```python
from build123d import *

# Parameters (mm, degrees)
SKETCH_1_W          = 32
SKETCH_1_H          = 10
EXTRUDE_1_DEPTH     = 4.5
SKETCH_2_R          = 2.1
CUT_EXTRUDE_1_DEPTH = 34.826764551
EXTRUDE_2_DEPTH     = 4
CHAMFER_1_SIZE      = 3
SKETCH_5_R          = 1.1
CUT_EXTRUDE_2_DEPTH = 34.826764551


with BuildPart() as part:
    # Эскиз1 → Бобышка-Вытянуть1 (new body)
    with BuildSketch(Plane.XY):
        with Locations((16, 5)):
            Rectangle(SKETCH_1_W, SKETCH_1_H)
    extrude(amount=EXTRUDE_1_DEPTH)

    # Эскиз2 → Вырез-Вытянуть1 (cut, through all)
    with BuildSketch(Plane(origin=(0, 10, 0), x_dir=(1, 0, 0), z_dir=(0, 1, 0))):
        with Locations((8.575, -5)):
            Circle(SKETCH_2_R)
        with Locations((23.425, -5)):
            Circle(SKETCH_2_R)
    extrude(amount=-CUT_EXTRUDE_1_DEPTH, mode=Mode.SUBTRACT)

    # Эскиз4 → Бобышка-Вытянуть2 (add)
    with BuildSketch(Plane.XZ.offset(-6)):
        with BuildLine():
            Line((6.535392195, 4.5), (7.055131585, 4.5))
            ThreePointArc((7.055131585, 4.5), (8.575, 3.4), (10.094868415, 4.5))
            Line((10.094868415, 4.5), (10.614607805, 4.5))
            ThreePointArc((10.614607805, 4.5), (8.575, 2.9), (6.535392195, 4.5))
        make_face()
        with BuildLine():
            Line((21.385392195, 4.5), (21.905131585, 4.5))
            ThreePointArc((21.905131585, 4.5), (23.425, 3.4), (24.944868415, 4.5))
            Line((24.944868415, 4.5), (25.464607805, 4.5))
            ThreePointArc((25.464607805, 4.5), (23.425, 2.9), (21.385392195, 4.5))
        make_face()
    extrude(amount=EXTRUDE_2_DEPTH)

    # Фаска1
    chamfer_1_edges = [part.edges().sort_by_distance(p)[0] for p in [
        (0, 5, 0),
        (32, 5, 0),
    ]]
    chamfer(chamfer_1_edges, length=CHAMFER_1_SIZE)

    # Эскиз5 → Вырез-Вытянуть2 (cut, through all)
    with BuildSketch(Plane(origin=(0, 0, 0), x_dir=(-1, 0, 0), z_dir=(0, 0, -1))):
        with Locations((-28.5, 5)):
            Circle(SKETCH_5_R)
        with Locations((-16, 5)):
            Circle(SKETCH_5_R)
        with Locations((-3.5, 5)):
            Circle(SKETCH_5_R)
    extrude(amount=-CUT_EXTRUDE_2_DEPTH, mode=Mode.SUBTRACT)

    # Фаска2: read off the stored shape, not the designer's step
    # Фаска2: loft between two sections, ruled curve by curve
    chamfer_2_from = [
        Edge.make_three_point_arc((3.288461538, 6.079468146, 1.5), (4.579468146, 5.211538462, 1.5), (3.711538462, 3.920531854, 1.5)),
        Edge.make_three_point_arc((3.711538462, 3.920531854, 1.5), (2.420531854, 4.788461538, 1.5), (3.288461538, 6.079468146, 1.5)),
    ]
    chamfer_2_to = [
        Edge.make_three_point_arc((2.999999479, 7.551472823, -2.709e-06), (6.051472823, 5.500000521, -2.709e-06), (4.000000521, 2.448527177, -2.709e-06)),
        Edge.make_three_point_arc((4.000000521, 2.448527177, -2.709e-06), (0.948527177, 4.499999479, -2.709e-06), (2.999999479, 7.551472823, -2.709e-06)),
    ]
    chamfer_2 = Solid(Shell([*[Face.make_surface_from_curves(chamfer_2_from[k], chamfer_2_to[k]) for k in range(2)], Face(Wire(chamfer_2_from)), Face(Wire(chamfer_2_to))]))
    add(chamfer_2, mode=Mode.SUBTRACT)

    # Chamfer 2 2: loft between two sections, ruled curve by curve
    chamfer_2_2_from = [
        Edge.make_three_point_arc((17.1, 5, 1.5), (16, 3.9, 1.5), (14.9, 5, 1.5)),
        Edge.make_three_point_arc((14.9, 5, 1.5), (16, 6.1, 1.5), (17.1, 5, 1.5)),
    ]
    chamfer_2_2_to = [
        Edge.make_three_point_arc((18.6, 5, 0), (16, 2.4, 0), (13.4, 5, 0)),
        Edge.make_three_point_arc((13.4, 5, 0), (16, 7.6, 0), (18.6, 5, 0)),
    ]
    chamfer_2_2 = Solid(Shell([*[Face.make_surface_from_curves(chamfer_2_2_from[k], chamfer_2_2_to[k]) for k in range(2)], Face(Wire(chamfer_2_2_from)), Face(Wire(chamfer_2_2_to))]))
    add(chamfer_2_2, mode=Mode.SUBTRACT)

    # Chamfer 2 3: loft between two sections, ruled curve by curve
    chamfer_2_3_from = [
        Edge.make_three_point_arc((28.711538462, 3.920531854, 1.5), (27.420531854, 4.788461538, 1.5), (28.288461538, 6.079468146, 1.5)),
        Edge.make_three_point_arc((28.288461538, 6.079468146, 1.5), (29.579468146, 5.211538462, 1.5), (28.711538462, 3.920531854, 1.5)),
    ]
    chamfer_2_3_to = [
        Edge.make_three_point_arc((29.000000521, 2.448527177, -2.709e-06), (25.948527177, 4.499999479, -2.709e-06), (27.999999479, 7.551472823, -2.709e-06)),
        Edge.make_three_point_arc((27.999999479, 7.551472823, -2.709e-06), (31.051472823, 5.500000521, -2.709e-06), (29.000000521, 2.448527177, -2.709e-06)),
    ]
    chamfer_2_3 = Solid(Shell([*[Face.make_surface_from_curves(chamfer_2_3_from[k], chamfer_2_3_to[k]) for k in range(2)], Face(Wire(chamfer_2_3_from)), Face(Wire(chamfer_2_3_to))]))
    add(chamfer_2_3, mode=Mode.SUBTRACT)


solid = part.part
```
Input: part model. Units: mm. Frame: model coordinates. A direction names the side the tool comes from. Give positions to 0.01 mm unless a question says otherwise; leave off trailing zeros. Order: outer loops, then holes, each group sorted by start corner. A loop starts at its lowest first (then second) coordinate and runs counter-clockwise, first axis right, second up. Notation, with made-up numbers: M 49,11.25 L 86,11.25 A25 ccw 86,40.25 Z; hole C -9,38.25 d9. An arc over 180 degrees is marked long. Return JSON: item names as keys, results as strings.
Item 1: Cut plane B-B (y = 1). Return loops of the section in (x, z) (3 decimals).
Solutions:
{"outline": "M 0,3 L 3,0 L 29,0 L 32,3 L 32,4.5 L 25.465,4.5 A2.1 cw 21.385,4.5 L 10.615,4.5 A2.1 cw 6.535,4.5 L 0,4.5 Z"}
Item 2: Ray query, probe 1 along X at (y, z) = (5, 3.1); probe 2 along Y at (x, z) = (3.5, 2.6); probe 3 along X at (y, z) = (4.75, 1.2). Return the intervals inside material, ascending.
Solutions:
{"probe 1": "0 to 2.4, 4.6 to 14.9, 17.1 to 27.4, 29.6 to 32", "probe 2": "0 to 3.9, 6.1 to 10", "probe 3": "1.8 to 2.12, 4.88 to 14.62, 17.38 to 27.12, 29.88 to 30.2"}
Item 3: Cut plane D-D (x = 9). Return loops of the section in (y, z).
Solutions:
{"outline": "M 0,0 L 10,0 L 10,2.94 L 6,2.94 L 6,3.46 L 2,3.46 L 2,2.94 L 0,2.94 Z"}
Item 4: Cut plane C-C (z = 1.8). Return loops of the section in (x, y), then the cut area to 3 significant figures.
Solutions:
{"outline": "M 1.2,0 L 30.8,0 L 30.8,10 L 1.2,10 Z; hole C 3.5,5 d2.2; hole C 16,5 d2.2; hole C 28.5,5 d2.2", "area": "285 mm^2"}
Item 5: Cut plane A-A (z = 3.7). State how many separate pieces and enclosed holes the cut face has, then the cut area to 3 significant figures.
Solutions:
{"separate pieces": "3", "enclosed holes": "3", "area": "254 mm^2"}
Item 6: First-contact query: P1, Ø3.5, axis at x = 28.5, y = 5, coming from the -Z side; P2, Ø0.5, axis at x = 23, z = 3.5, coming from the -Y side; P3, Ø1.3, axis at x = 9, z = 4, coming from the +Y side. Flat tips, straight axial feed; report the tip coordinate or a pass-through.
Solutions:
{"P1": "z = 0.85", "P2": "y = 2", "P3": "y = 6"}
Item 7: Pull-direction query (X, two-part tool) for faces 4 (the flat face through (31, 5, 2)), 5 (the cylindrical face through (2.484, 4.579, 2.979)), 6 (the flat face through (16, 10, 2)); classes: +X half, -X half, draft (parallel to the pull), parting line (faces both ways), or undercut.
Solutions:
{"face 4": "+X half", "face 5": "undercut", "face 6": "draft"}
Item 8: Access query for faces 1 (the cylindrical face through (8.6, 1, 2.9)), 2 (the flat face through (8.4, 6, 3.2)), 3 (the flat face through (14.6, 5.1, 4.5)). Directions: +Z, -Z, +X, -X, +Y, -Y. A direction counts if a zero-diameter tool reaches every point of the face in a straight line with its end or side. Return the directions, or none.
Solutions:
{"face 1": "+Z, -Y", "face 2": "+Z, +Y", "face 3": "+Z, +X, -X, +Y, -Y"}
